from build123d import *

# Parameters (mm, degrees)
SKETCH1_R           = 1.862815958
SKETCH1_R_2         = 1.6
BOSS_EXTRUDE1_DEPTH = 3


with BuildPart() as part:
    # Sketch1 → Boss-Extrude1 (new body)
    with BuildSketch(Plane(origin=(0, 0, 0), x_dir=(0, 0, -1), z_dir=(1, 0, 0))):
        with BuildLine():
            Line((40, 6), (0, 6))
            ThreePointArc((0, 6), (-6, 0), (0, -6))
            Line((0, -6), (40, -6))
            Line((40, -6), (40, 6))
        make_face()
        with Locations((25, -1)):
            Circle(SKETCH1_R, mode=Mode.SUBTRACT)
        with Locations((35, -1)):
            Circle(SKETCH1_R_2, mode=Mode.SUBTRACT)
        Circle(SKETCH1_R_2, mode=Mode.SUBTRACT)
    extrude(amount=BOSS_EXTRUDE1_DEPTH)


solid = part.part
Design review of the part built by this model. Coordinates are the model's own, in mm. Give positions to 0.01 mm unless a question says otherwise; leave off trailing zeros. Order: outer loops, then holes, each group sorted by start corner. A loop starts at its lowest first (then second) coordinate and runs counter-clockwise, first axis right, second up. Notation, with made-up numbers: (35, 56) - (86, 56) arc R9 cw to (86, 60) - close; hole circle Ø3 at (80, -3). An arc over 180 degrees is marked (long way). Write item = value, one per line. Start each with the question number.
Q1. Mouldability with a two-part tool opening along Y and no side actions: class faces 1 (the face through (1.479, -1.713, -26.721)), 2 (the face through (1.48, -0.97, 1.27)), 3 (the face through (0, 0, -17)), 4 (the face through (1, -6, -20)) as released by +Y, released by -Y, zero draft, split by the parting line, or undercut.
Q2. Clearance check with a flat-ended pin moving along its axis: pin 1 Ø3 at (y, z) = (0, 0) entering from +X. State where the tip first meets the part, or that it passes through.
Q3. We need section D-D on z = -35. State the section outline as (x, y) points.
Q4. We need section A-A on z = -25. State the section outline as (x, y) points, plus the area to 3 significant figures.
Q5. We need section B-B on x = 1. State the section outline as (y, z) points.
Q6. We need section C-C on y = 0. State the section outline as (x, z) points, plus the area to 3 significant figures.
Q7. To check wall thickness, follow L1, parallel to Y at x = 1, z = 0; L2, parallel to Y at x = 1.4, z = -25; L3, parallel to Z at x = 1.8, y = 1. State the ranges of each line that lie inside material, in increasing order. Write a range as from..to.
Working result:
q1.face_1 = undercut
q1.face_2 = undercut
q1.face_3 = zero draft
q1.face_4 = released by -Y
q2.pin_1 = through
q3.outline = (0, -6) - (3, -6) - (3, -2.6) - (0, -2.6) - close; (0, 0.6) - (3, 0.6) - (3, 6) - (0, 6) - close
q4.outline = (0, -6) - (3, -6) - (3, -2.86) - (0, -2.86) - close; (0, 0.86) - (3, 0.86) - (3, 6) - (0, 6) - close
q4.area = 24.8 mm²
q5.outline = (-6, -40) - (6, -40) - (6, 0) arc R6 ccw to (-6, 0) - close; hole circle Ø3.73 at (-1, -25); hole circle Ø3.2 at (-1, -35); hole circle Ø3.2 at (0, 0)
q6.outline = (0, -40) - (3, -40) - (3, -36.25) - (0, -36.25) - close; (0, -33.75) - (3, -33.75) - (3, -26.57) - (0, -26.57) - close; (0, -23.43) - (3, -23.43) - (3, -1.6) - (0, -1.6) - close; (0, 1.6) - (3, 1.6) - (3, 6) - (0, 6) - close
q6.area = 111 mm²
q7.L1 = -6..-1.6, 1.6..6
q7.L2 = -6..-2.86, 0.86..6
q7.L3 = -40..-1.25, 1.25..5.92
